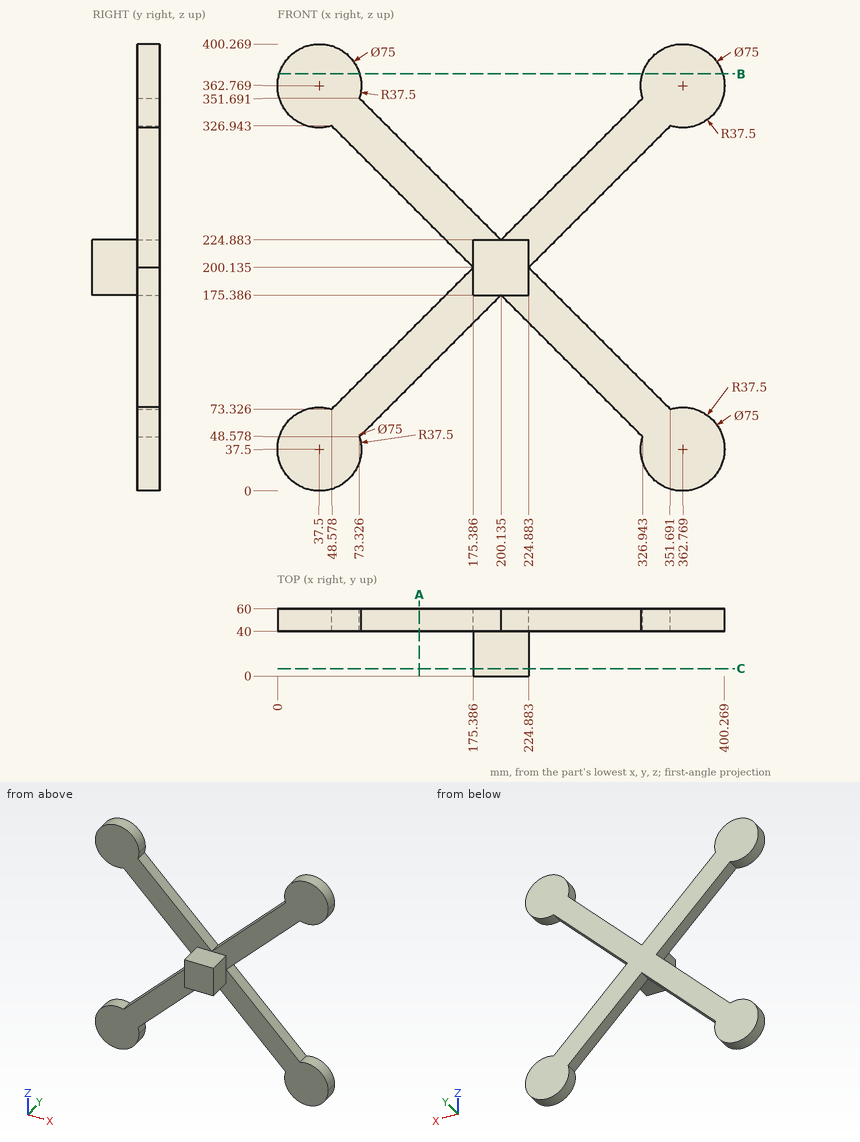
Study the drawing (mm; zero at the part's minimum x, y, z) and answer. Coordinates: 2 decimals unless noted, no trailing zeros. Write each loop counter-clockwise with the first axis right and the second up, starting at its lowest first coordinate (ties: lowest second). Pieces come first, ordered by that corner, then holes. Notation, with made-up numbers: (5.5, -36.75) - (57.5, -36.75) arc R22 ccw to (57.5, -26.75) - close; hole circle Ø1 at (-4, 82.25). An arc over 180 degrees is marked (long way). Answer as a JSON object with one key per item and string values. Group by question number.
1. Each of these flat-tipped pins is pushed along its axis until it touches: P1, Ø6, axis at y = 42, z = 256, coming from the +X side; P2, Ø12, axis at y = 39, z = 151.5, coming from the +X side (1 decimal); P3, Ø8, axis at y = 35.5, z = 296, coming from the -X side; P4, Ø20, axis at y = 28.5, z = 206.5, coming from the +X side. Where does it stop, or does it pass through?
2. Consider L1, parallel to Z at x = 16.5, y = 53.5; L2, parallel to X at y = 50, z = 295; L3, parallel to Z at x = 113.5, y = 52.5. Determine where each line is inside the solid, lowest interval first. Write a range as [from, to].
3. A cutting plane is placed at C-C (y = 6.5). Determine the outline of the cut face in (x, z) (1 decimal), plus the area to 3 significant figures.
4. A cutting plane is placed at A-A (x = 127). Determine the outline of the cut face in (y, z).
5. A cutting plane is placed at B-B (z = 373.5). Determine the outline of the cut face in (x, y), plus the area to 3 significant figures.
Worked out:
{
 "1": {"P1": "stops at x = 283.75", "P2": "stops at x = 279.4", "P3": "passes through", "P4": "stops at x = 224.88"},
 "2": {"L1": "z = [6.43, 68.57], [331.7, 393.84]", "L2": "x = [80.52, 130.02], [270.25, 319.75]", "L3": "z = [88.75, 138.25], [262.02, 311.52]"},
 "3": {"outline": "(175.4, 175.4) - (224.9, 175.4) - (224.9, 224.9) - (175.4, 224.9) - close", "area": "2,450 mm²"},
 "4": {"outline": "(40, 102.25) - (60, 102.25) - (60, 151.75) - (40, 151.75) - close; (40, 248.52) - (60, 248.52) - (60, 298.02) - (40, 298.02) - close"},
 "5": {"outline": "(1.57, 40) - (73.43, 40) - (73.43, 60) - (1.57, 60) - close; (326.84, 40) - (398.7, 40) - (398.7, 60) - (326.84, 60) - close", "area": "2,870 mm²"}
}
